The model under review builds one solid part; all positions refer to its coordinate system, in mm. A direction names the side the tool comes from. Round coordinates to 2 decimals unless told otherwise and drop trailing zeros. Write each loop counter-clockwise with the first axis right and the second up, starting at its lowest first coordinate (ties: lowest second). Pieces come first, ordered by that corner, then holes. Notation, with made-up numbers: (-2, 42) -> (52, 42) arc R17 cw to (52, 49) -> close; hole circle Ø1 at (34, 7). An arc over 180 degrees is marked (long way). Answer as a JSON object with one key per item and string values. Group by question number.
1) Machinability: for faces 1 (the cylindrical face through (-1.08, -4.88, 32.11)), 2 (the flat face through (-6, 0, -10)), which of the approach directions +Z, -Z, +X, -X, +Y, -Y give a long, thin tool a straight path to every point of the face, cutting with its end or side? Answer none if there is none.
2) We need section D-D, the plane x = 6.5. Write out the cut boundary in (y, z).
3) We need section C-C, the plane z = 51.5. Write out the cut boundary in (x, y), then the cut area to 3 significant figures.
4) We need section B-B, the plane y = 1.5. Write out the cut boundary in (x, z), then the cut area to 3 significant figures.
5) To check wall thickness, follow probe 1 along Y at (x, z) = (0, -7); probe 2 along Z at (x, y) = (-6, -6.5); probe 3 along Y at (x, z) = (2.75, 3.5). State the ranges of each line that lie inside material, in increasing order. Write a range as [from, to].
6) Insertion check: pin 1 Ø2 at (x, y) = (-3.5, 1) entering from -Z; pin 2 Ø8 at (x, z) = (5, 7) entering from -Y; pin 3 Ø5 at (y, z) = (-1, 31) entering from +X; pin 4 Ø13 at (x, y) = (-6, -6) entering from +Z. Each pin has a flat end and moves straight along its axis. Give the tip position at first contact, or say it passes through.
7) We need section A-A, the plane x = 0. Write out the cut boundary in (y, z), then the cut area to 3 significant figures.
8) Mouldability with a two-part tool opening along Y and no side actions: class faces 3 (the cylindrical face through (10.316, -7.91, -2.395)), 4 (the flat face through (0, 0, 60)), 5 (the flat face through (0, 0, 0)), 6 (the cylindrical face through (1.08, -4.88, -5.07)) as pulls with the +Y half, pulls with the -Y half, needs draft (parallel to the pull), parting line crosses it, or undercut.
from build123d import *

# Parameters (mm, degrees)
SKETCH1_R           = 5
BOSS_EXTRUDE1_DEPTH = 60
SKETCH2_R           = 13
BOSS_EXTRUDE2_DEPTH = 15
SKETCH3_R           = 5
CUT_EXTRUDE2_DEPTH  = 10


with BuildPart() as part:
    # Sketch1 → Boss-Extrude1 (new body)
    with BuildSketch(Plane.XY):
        Circle(SKETCH1_R)
    extrude(amount=BOSS_EXTRUDE1_DEPTH)

    # Sketch2 → Boss-Extrude2 (add)
    with BuildSketch(Plane(origin=(0, 0, 5), x_dir=(-1, 0, 0), z_dir=(0, 0, -1))):
        Circle(SKETCH2_R)
    extrude(amount=BOSS_EXTRUDE2_DEPTH)

    # Sketch3 → Cut-Extrude2 (cut)
    with BuildSketch(Plane(origin=(0, 0, -10), x_dir=(-1, 0, 0), z_dir=(0, 0, -1))):
        Circle(SKETCH3_R)
    extrude(amount=-CUT_EXTRUDE2_DEPTH, mode=Mode.SUBTRACT)


solid = part.part
Here are the results:
{
 "1": {"face 1": "+Z", "face 2": "-Z, +X, -X, +Y, -Y"},
 "2": {"outline": "(-11.26, -10) -> (11.26, -10) -> (11.26, 5) -> (-11.26, 5) -> close"},
 "3": {"outline": "circle Ø10 at (0, 0)", "area": "78.5 mm^2"},
 "4": {"outline": "(-12.91, -10) -> (-4.77, -10) -> (-4.77, 0) -> (4.77, 0) -> (4.77, -10) -> (12.91, -10) -> (12.91, 5) -> (4.77, 5) -> (4.77, 60) -> (-4.77, 60) -> (-4.77, 5) -> (-12.91, 5) -> close", "area": "817 mm^2"},
 "5": {"probe 1": "y = [-13, -5], [5, 13]", "probe 2": "z = [-10, 5]", "probe 3": "y = [-12.71, 12.71]"},
 "6": {"pin 1": "stops at z = 0", "pin 2": "stops at y = -12.91", "pin 3": "stops at x = 5", "pin 4": "stops at z = 60"},
 "7": {"outline": "(-13, -10) -> (-5, -10) -> (-5, 0) -> (5, 0) -> (5, -10) -> (13, -10) -> (13, 5) -> (5, 5) -> (5, 60) -> (-5, 60) -> (-5, 5) -> (-13, 5) -> close", "area": "840 mm^2"},
 "8": {"face 3": "parting line crosses it", "face 4": "needs draft", "face 5": "undercut", "face 6": "undercut"}
}
